Verification items for this drawing (mm, ordinates from the low corner). A direction names the side the tool comes from. Round coordinates to 2 decimals unless told otherwise and drop trailing zeros. Write each loop counter-clockwise with the first axis right and the second up, starting at its lowest first coordinate (ties: lowest second). Pieces come first, ordered by that corner, then holes. Notation, with made-up numbers: (-21, 77.25) -> (12, 77.25) arc R18 ccw to (12, 96.25) -> close; hole circle Ø8 at (-40, -7.75). An arc over 180 degrees is marked (long way). Put each result on its own line as item: value. Start each with the question number.
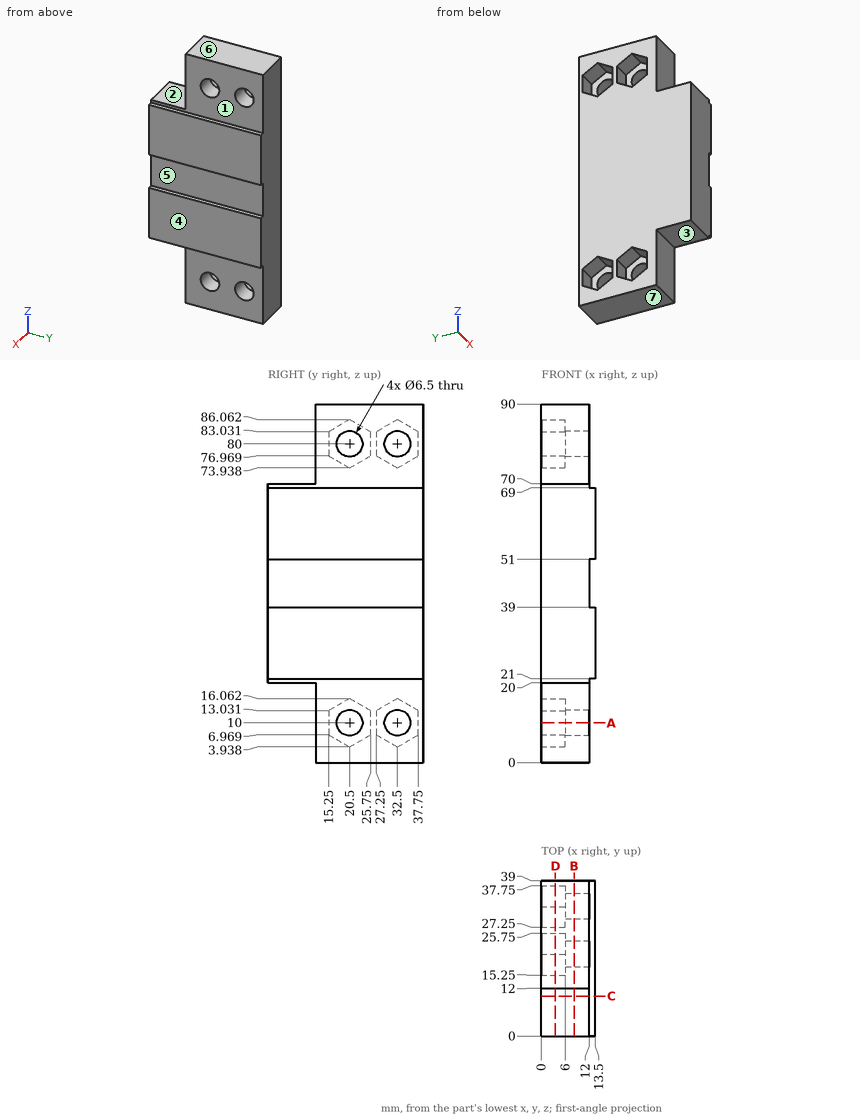
(1) Sectioned sample at A-A (z = 10). Record the cut outline in (x, y), and give its area (3 significant figures).
(2) Sectioned sample at C-C (y = 10). Record the cut outline in (x, z).
(3) Sectioned sample at D-D (x = 3.5). State how many separate pieces and enclosed holes the cut face has, and give its area (3 significant figures).
(4) Set-up check for the marked faces 1, 2 and 3: record each of +Z, -Z, +X, -X, +Y, -Y from which the full face is reachable in a straight line by a thin tool's end or side.
(5) Sectioned sample at B-B (x = 8.25). Record the cut outline in (y, z).
(6) Mould release check, pull along Z, two halves, no side actions. Record for the marked faces 4, 5, 6 and 7: +Z half, -Z half, draft (parallel to the pull), parting line (faces both ways), or undercut.
(7) Go/stop test with flat-tipped pins: pin 1 Ø10.5 at (y, z) = (11, 81) entering from +X; pin 2 Ø1.5 at (x, y) = (7, 7) entering from -Z; pin 3 Ø1.2 at (x, y) = (13, 25) entering from -Z; pin 4 Ø6 at (y, z) = (20.5, 80) entering from -X. Record where each tip stops, or that it passes through.
(8) Material ranges on L1, parallel to Y at x = 7.5, z = 80; L2, parallel to Z at x = 5, y = 28; L3, parallel to Z at x = 8.25, y = 22, recorded low to high. Write a range as from..to.
Found:
1. outline: (0, 12) -> (12, 12) -> (12, 17.25) -> (6, 17.25) -> (6, 15.25) -> (0, 15.25) -> close; (0, 25.75) -> (6, 25.75) -> (6, 23.75) -> (12, 23.75) -> (12, 29.25) -> (6, 29.25) -> (6, 27.25) -> (0, 27.25) -> close; (0, 37.75) -> (6, 37.75) -> (6, 35.75) -> (12, 35.75) -> (12, 39) -> (0, 39) -> close
1. area: 120 mm2
2. outline: (0, 20) -> (12, 20) -> (12, 21) -> (13.5, 21) -> (13.5, 39) -> (12, 39) -> (12, 51) -> (13.5, 51) -> (13.5, 69) -> (12, 69) -> (12, 70) -> (0, 70) -> close
3. separate pieces: 1
3. enclosed holes: 4
3. area: 2,650 mm2
4. face 1: +Z, +X, +Y, -Y
4. face 2: +Z, +X, -X, -Y
4. face 3: -Z, +X, -X, -Y
5. outline: (0, 20) -> (12, 20) -> (12, 0) -> (39, 0) -> (39, 90) -> (12, 90) -> (12, 70) -> (0, 70) -> close; hole circle Ø6.5 at (20.5, 10); hole circle Ø6.5 at (20.5, 80); hole circle Ø6.5 at (32.5, 10); hole circle Ø6.5 at (32.5, 80)
6. face 4: draft
6. face 5: undercut
6. face 6: +Z half
6. face 7: -Z half
7. pin 1: x = 12
7. pin 2: z = 20
7. pin 3: z = 21
7. pin 4: through
8. L1: 12..17.25, 23.75..29.25, 35.75..39
8. L2: 0..6.54, 13.46..76.54, 83.46..90
8. L3: 0..7.12, 12.88..77.12, 82.88..90
